from build123d import *

# Parameters (mm, degrees)
SKETCH1_R               = 12.6
BOSS_EXTRUDE1_DEPTH     = 1
CUT_EXTRUDE4_DEPTH      = 18.847128621
CUT_EXTRUDE4_DEPTH_BACK = 18.847128621
FILLET1_R               = 1


with BuildPart() as part:
    # Sketch1 → Boss-Extrude1 (new body)
    with BuildSketch(Plane(origin=(0, 0, 0), x_dir=(1, 0, 0), z_dir=(0, 1, 0))):
        with Locations(Location((0, 0, 0), (0, 0, 270))):
            Circle(SKETCH1_R)
    extrude(amount=BOSS_EXTRUDE1_DEPTH)

    # Sketch2 → Cut-Extrude4 (cut, two sides: drawn at the far end of the back side and taken through both)
    with BuildSketch(Plane(origin=(0, 0, 0), x_dir=(1, 0, 0), z_dir=(0, 1, 0)).offset(-CUT_EXTRUDE4_DEPTH_BACK)):
        with BuildLine():
            Line((-6.1, 0), (-6.1, 13.442202198))
            ThreePointArc((-6.1, 13.442202198), (0, 19.542202198), (6.1, 13.442202198))
            Line((6.1, 13.442202198), (6.1, 0))
            ThreePointArc((6.1, 0), (0, -6.1), (-6.1, 0))
        make_face()
    extrude(amount=CUT_EXTRUDE4_DEPTH + CUT_EXTRUDE4_DEPTH_BACK, mode=Mode.SUBTRACT)

    # Fillet1
    fillet1_edges = [part.edges().sort_by_distance(p)[0] for p in [
        (6.1, 0.5, -11.024971655),
        (-6.1, 0.5, -11.024971655),
    ]]
    fillet(fillet1_edges, radius=FILLET1_R)


solid = part.part
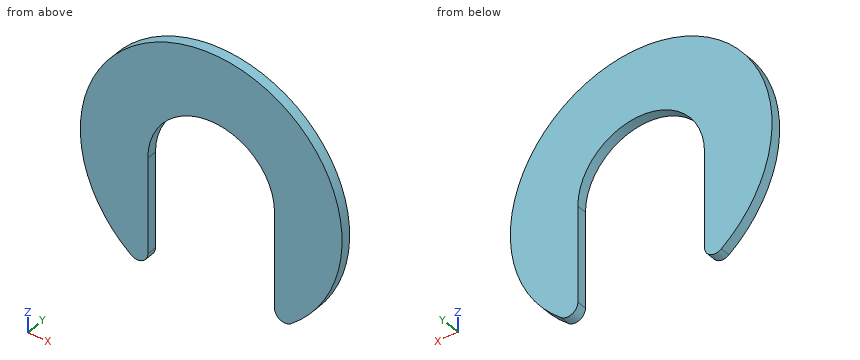
Source: CAD feature listing. Evaluate the final solid. Frame: model axes, mm. Give positions to 0.01 mm unless a question says otherwise; leave off trailing zeros. Write each loop counter-clockwise with the first axis right and the second up, starting at its lowest first coordinate (ties: lowest second). Pieces come first, ordered by that corner, then holes. Notation, with made-up numbers: (-39.5, -0.5) - (-2.5, -0.5) arc R21 cw to (-2.5, 3.5) - close; hole circle Ø4 at (65.5, -4.75). An arc over 180 degrees is marked (long way). Write item = value, one per line. Start each with the question number.
Q1. Cut plane A-A, the plane z = -8.5. Return loops of the section in (x, y), then the cut area to 3 significant figures.
Q2. Cut plane D-D, the plane x = 0. Return loops of the section in (y, z).
Q3. Cut plane C-C, the plane z = 4. Return loops of the section in (x, y), then the cut area to 3 significant figures.
Q4. Cut plane B-B, the plane y = 0.65. Return loops of the section in (x, z).
Q5. Pin query (flat end, axial travel): pin 1 Ø1.5 at (x, z) = (-5.5, 2) entering from +Y; pin 2 Ø0.5 at (y, z) = (0.5, -6) entering from +X. Return the tip coordinate at first contact, or that it passes through.
Q6. Material intervals for probe 1 along X at (y, z) = (0.65, -2); probe 2 along X at (y, z) = (0.65, 5); probe 3 along Z at (x, y) = (-0.25, 0.85), sorted ascending.
Computed values:
q1.outline = (-9.3, 0) - (-6.1, 0) - (-6.1, 1) - (-9.3, 1) - close; (6.1, 0) - (9.3, 0) - (9.3, 1) - (6.1, 1) - close
q1.area = 6.40 mm²
q2.outline = (0, 6.1) - (1, 6.1) - (1, 12.6) - (0, 12.6) - close
q3.outline = (-11.95, 0) - (-4.61, 0) - (-4.61, 1) - (-11.95, 1) - close; (4.61, 0) - (11.95, 0) - (11.95, 1) - (4.61, 1) - close
q3.area = 14.7 mm²
q4.outline = (-7.71, -9.96) arc R1 ccw to (-6.1, -9.17) - (-6.1, 0) arc R6.1 cw to (6.1, 0) - (6.1, -9.17) arc R1 ccw to (7.71, -9.96) arc R12.6 ccw (long way) to start
q5.pin_1 = 1
q5.pin_2 = 11.21
q6.probe_1 = -12.44 to -6.1, 6.1 to 12.44
q6.probe_2 = -11.57 to -3.49, 3.49 to 11.57
q6.probe_3 = 6.09 to 12.6
